from build123d import *

# Parameters (mm, degrees)
SKETCH3_R           = 60.325
BOSS_EXTRUDE1_DEPTH = 8.89
CHAMFER1_SIZE       = 12.7
CHAMFER1_SIZE_2     = 6.35
CUT_EXTRUDE1_DEPTH  = 3.81
FILLET1_R           = 3.81
CIRPATTERN1_START   = 38.301794875
CIRPATTERN1_DEPTH   = 3.81
SKETCH5_R           = 8
BOSS_EXTRUDE2_DEPTH = 60


# Read off the part's stored shape, not the designer's step: CirPattern1
with BuildPart() as part:
    # Sketch1 → Revolve1 (revolve)
    with BuildSketch(Plane.XZ, mode=Mode.PRIVATE) as revolve1_sk:
        with BuildLine():
            ThreePointArc((-33.221794875, -65.71974362), (0, -81.28), (33.221794875, -65.71974362))
            Line((33.221794875, -65.71974362), (33.221794875, 0))
            Line((33.221794875, 0), (-33.221794875, 0))
            Line((-33.221794875, 0), (-33.221794875, -65.71974362))
        make_face()
    revolve(revolve1_sk.sketch.rotate(Axis((-33.221794875, 0, 0), (1, 0, 0)), 180), axis=Axis((-33.221794875, 0, 0), (1, 0, 0)))

    # Sketch3 → Boss-Extrude1 (add)
    with BuildSketch(Plane(origin=(33.221794875, 0, 0), x_dir=(0, 0, -1), z_dir=(1, 0, 0))):
        with Locations(Location((0, 0, 0), (0, 0, 180))):
            Circle(SKETCH3_R)
    extrude(amount=BOSS_EXTRUDE1_DEPTH)

    # Chamfer1
    # the kernel refuses this chamfer: 12.7, 6.35 mm, written as the material it takes off along each edge
    with BuildSketch(Plane(origin=(42.111794875, 0, 0), x_dir=(0, 0, 1), z_dir=(0, 1, 0))) as chamfer1_piece_1_section:
        Polygon((60.325, -CHAMFER1_SIZE), (60.325 - CHAMFER1_SIZE_2, 0), (60.325, 0), align=None)
    chamfer1_piece_1 = revolve(axis=Axis((42.111794875, 0, 0), (1, 0, 0)), mode=Mode.PRIVATE)
    chamfer1_piece_1 = split(chamfer1_piece_1, bisect_by=Plane(origin=(33.221794875, 0, -56.304392735), z_dir=(1, 0, 0)), keep=Keep.TOP, mode=Mode.PRIVATE)
    add(chamfer1_piece_1, mode=Mode.SUBTRACT)

    # Sketch4 → Cut-Extrude1 (cut)
    with BuildSketch(Plane(origin=(42.111794875, 0, 0), x_dir=(0, 0, -1), z_dir=(1, 0, 0))):
        with BuildLine():
            ThreePointArc((-3.287001873, 12.267257994), (0, -12.7), (3.287001873, 12.267257994))
            Line((3.287001873, 12.267257994), (12.983657398, 48.455669076))
            ThreePointArc((12.983657398, 48.455669076), (0, 50.165), (-12.983657398, 48.455669076))
            Line((-12.983657398, 48.455669076), (-3.287001873, 12.267257994))
        make_face()
    extrude(amount=-CUT_EXTRUDE1_DEPTH, mode=Mode.SUBTRACT)

    # Fillet1
    fillet1_edges = [part.edges().sort_by_distance(p)[0] for p in [
        (40.206794875, 48.455669076, -12.983657398),
        (40.206794875, 12.267257994, 3.287001873),
        (40.206794875, 48.455669076, 12.983657398),
        (40.206794875, 12.267257994, -3.287001873),
    ]]
    fillet(fillet1_edges, radius=FILLET1_R)

    # CirPattern1 outline → CirPattern1 (cut)
    with BuildSketch(Plane.YZ.offset(CIRPATTERN1_START)):
        with BuildLine():
            ThreePointArc((-29.073443692, 35.902712946), (-31.792302862, 37.307304663), (-34.667331707, 36.258838058))
            ThreePointArc((-34.667331707, 36.258838058), (-40.584337523, 29.486247181), (-45.196998855, 21.765994566))
            ThreePointArc((-45.196998855, 21.765994566), (-45.30571708, 18.70768565), (-43.129697286, 16.55593963))
            Line((-43.129697286, 16.55593963), (-11.856471417, 4.551272959))
            ThreePointArc((-11.856471417, 4.551272959), (-10.274515829, 7.464872704), (-7.992368966, 9.869753711))
            Line((-7.992368966, 9.869753711), (-29.073443692, 35.902712946))
        make_face()
        with BuildLine():
            Line((2.417824845, 46.134846353), (0.664666644, 12.682595091))
            ThreePointArc((0.664666644, 12.682595091), (3.924515829, 12.078417757), (6.916915745, 10.651116213))
            Line((6.916915745, 10.651116213), (25.161320914, 38.745036519))
            ThreePointArc((25.161320914, 38.745036519), (25.656993331, 41.764867961), (23.771409561, 44.175188879))
            ThreePointArc((23.771409561, 44.175188879), (15.501837523, 47.70975014), (6.734050225, 49.710962499))
            ThreePointArc((6.734050225, 49.710962499), (3.791829822, 48.869290246), (2.417824845, 46.134846353))
        make_face()
        with BuildLine():
            ThreePointArc((6.916915745, -10.651116213), (3.924515829, -12.078417757), (0.664666644, -12.682595091))
            Line((0.664666644, -12.682595091), (2.417824845, -46.134846353))
            ThreePointArc((2.417824845, -46.134846353), (3.791829822, -48.869290246), (6.734050225, -49.710962499))
            ThreePointArc((6.734050225, -49.710962499), (15.501837523, -47.70975014), (23.771409561, -44.175188879))
            ThreePointArc((23.771409561, -44.175188879), (25.656993331, -41.764867961), (25.161320914, -38.745036519))
            Line((25.161320914, -38.745036519), (6.916915745, -10.651116213))
        make_face()
        with BuildLine():
            ThreePointArc((-7.992368966, -9.869753711), (-10.274515829, -7.464872704), (-11.856471417, -4.551272959))
            Line((-11.856471417, -4.551272959), (-43.129697286, -16.55593963))
            ThreePointArc((-43.129697286, -16.55593963), (-45.30571708, -18.70768565), (-45.196998855, -21.765994566))
            ThreePointArc((-45.196998855, -21.765994566), (-40.584337523, -29.486247181), (-34.667331707, -36.258838058))
            ThreePointArc((-34.667331707, -36.258838058), (-31.792302862, -37.307304663), (-29.073443692, -35.902712946))
            Line((-29.073443692, -35.902712946), (-7.992368966, -9.869753711))
        make_face()
    extrude(amount=CIRPATTERN1_DEPTH, mode=Mode.SUBTRACT)

    # Sketch5 → Boss-Extrude2 (add)
    with BuildSketch(Plane.ZY.offset(33.221794875)):
        with Locations(Location((0, 0, 0), (0, 0, 180))):
            Circle(SKETCH5_R)
    extrude(amount=BOSS_EXTRUDE2_DEPTH)


solid = part.part
Part model, mm, in its own coordinate system. A direction names the side the tool comes from. Coordinates: 2 decimals unless noted, no trailing zeros. Write each loop counter-clockwise with the first axis right and the second up, starting at its lowest first coordinate (ties: lowest second). Pieces come first, ordered by that corner, then holes. Notation, with made-up numbers: M 50.25,25 L 68.25,25 A15 ccw 68.25,50 Z; hole C 35,0.5 d10. An arc over 180 degrees is marked long. Return JSON: item names as keys, results as strings.
1. Probe L1, parallel to X at y = 43, z = 9.5; L2, parallel to X at y = 29, z = 45; L3, parallel to Y at x = -16, z = -42. List the from-to ranges inside material, lowest first.
Determined:
{"L1": "-33.22 to 38.3", "L2": "-33.22 to 42.11", "L3": "-65.98 to 65.98"}
2. Flat gauge pins, fed straight in: pin 1 Ø6 at (y, z) = (-61.5, 41) entering from -X; pin 2 Ø8 at (y, z) = (27.5, -62.5) entering from +X; pin 3 Ø4 at (x, z) = (20.5, -41.5) entering from +Y; pin 4 Ø6 at (x, y) = (-45, -11.5) entering from +Z. Where does each tip first touch, or does it go through?
Determined:
{"pin 1": "x = -28.09", "pin 2": "x = 33.22", "pin 3": "y = 65.56", "pin 4": "through"}
3. 3-axis set-ups, long thin cutter, end or side, ignore diameter. For faces 4 (the face through (40.23, 9.31, -8.64)), 5 (the face through (-93.222, 0, 0)): which of +Z, -Z, +X, -X, +Y, -Y reach the whole face in a straight line?
Determined:
{"face 4": "+X", "face 5": "+Z, -Z, -X, +Y, -Y"}
4. Saw through at A-A, the plane x = -76. Write the cut outline in (y, z), then the cut area to 3 significant figures.
Determined:
{"outline": "C 0,0 d16", "area": "201 mm²"}
5. Pull direction Y, two halves, no side cores. Call faces 1 (the face through (40.18, 15.62, 47.67)), 2 (the face through (-62.8, 7.81, 1.73)), 3 (the face through (42.112, -13, -1)): pulls with the +Y half, pulls with the -Y half, needs draft (parallel to the pull), parting line crosses it, or undercut.
Determined:
{"face 1": "undercut", "face 2": "parting line crosses it", "face 3": "needs draft"}
